Autodesk Inventor part; units mm, degrees
ref_plane "YZ Plane" through (0, 0, 0) normal (1, 0, 0) x (0, 1, 0)
ref_plane "XZ Plane" through (0, 0, 0) normal (0, 1, 0) x (-1, 0, 0)
ref_plane "XY Plane" through (0, 0, 0) normal (0, 0, 1) x (1, 0, 0)
sketch "Sketch1" plane through (0, 0, 0) normal (0, 1, 0) x (-1, 0, 0)
  line L0 (6, -3.4641) -> (0, -6.9282)
  line L1 (0, -6.9282) -> (-6, -3.4641)
  line L2 (-6, -3.4641) -> (-6, 3.4641)
  line L3 (-6, 3.4641) -> (0, 6.9282)
  line L4 (0, 6.9282) -> (6, 3.4641)
  line L5 (6, 3.4641) -> (6, -3.4641)
  circle A0 centre (0, 0) radius 2
  dimension "d0" = 6
  dimension "d1" = 4
extrude "Extrusion1" add sketch "Sketch1" along normal blind 6
sketch "Sketch2" plane through (0, 6, 0) normal (0, 1, 0) x (1, 0, 0)
  circle A0 centre (0, 0) radius 3
  circle A1 centre (0, 0) radius 5.5
  dimension "d4" = 6
  dimension "d5" = 11
extrude "Extrusion2" add sketch "Sketch2" along normal blind 12
sketch "Sketch3" plane through (0, 0, 0) normal (0, 0, 1) x (1, 0, 0)
  circle A0 centre (0, 15) radius 1.5
  line L0 (0, 0) -> (0, 6)
  line L1 (5.5, 18) -> (-5.5, 18)
  dimension "d16" = 3
  dimension "d44" = 0
  dimension "d45" = 3
extrude "Extrusion3" cut sketch "Sketch3" along normal mid plane 24
chamfer "Chamfer" distance 0.5 angle 45 4 edges at (2, 0, 0) (-3, 18, 0) (-1.5, 15.0054, -5.2915) (-1.5, 15.0054, 5.2915)
sketch "Sketch4" plane through (0, 0, 0) normal (1, 0, 0) x (0, 1, 0)
  line L0 (0, -3.4641) -> (0, -6.9282)
  line L1 (0, -6.9282) -> (0, -5.9282)
  line L2 (0, -6.9282) -> (1, -6.9282)
  line L3 (1, -6.9282) -> (0, -5.9282)
  line L4 (-6, 0) -> (36, 0)
  line L5 (0, -6.9282) -> (6, -6.9282)
  line L6 (6, -6.9282) -> (5, -6.9282)
  line L7 (6, -6.9282) -> (6, -5.9282)
  line L8 (6, -5.9282) -> (5, -6.9282)
  dimension "d31" = 1
  dimension "d32" = 1
  dimension "d36" = 1
  dimension "d37" = 1
revolve "Revolution" cut sketch "Sketch4" angle 360 about axis through (0, -10, 0) along (0, 1, 0)
thread "Thread1"
thread "Thread2"
thread "Thread3"
properties part number "6mmID_30mmL_hex_adapter"
Part model, mm, in its own coordinate system. A direction names the side the tool comes from. Coordinates: 2 decimals unless noted, no trailing zeros. Write each loop counter-clockwise with the first axis right and the second up, starting at its lowest first coordinate (ties: lowest second). Pieces come first, ordered by that corner, then holes.
Item 1: Mould opens along Z. For faces 3 (the face through (2.96, 2.96, -5.22)), 4 (the face through (1.61, 11.67, 2.53)), 5 (the face through (-4, 6, -4)), 6 (the face through (-1, 6, -2)) say: released by +Z, released by -Z, zero draft, split by the parting line, or undercut.
Item 2: Which spindle directions (+Z, -Z, +X, -X, +Y, -Y) get a long thin tool onto all of the face, cutting with end or side? Do faces 1 (the face through (1.43, 15.45, -3.78)), 2 (the face through (2.5, 11.9, -4.9)). Say none if no direction does.
Item 3: Slice it at C-C (x = -0.5). Count the separate pieces of the cut face and the enclosed holes in it, and give its area (3 significant figures).
Item 4: Pin check, flat tips, straight feed: pin 1 (3.5 mm diameter, centred on x = 0, z = 0, fed in from -Y); pin 2 (1.8 mm diameter, centred on x = 1, z = 1.5, fed in from +Y); pin 3 (1 mm diameter, centred on y = 7.5, z = -4, fed in from +X); pin 4 (5 mm diameter, centred on x = 2, y = 11.5, fed in from +Z). Stop position of each tip, or through.
Item 5: Slice it at B-B (y = 2.5). Write the cut outline in (x, z).
Item 6: Slice it at D-D (y = 11.5). Write the cut outline in (x, z), and give its area (3 significant figures).
Item 7: Slice it at A-A (z = 0). Write the cut outline in (x, y), and give its area (3 significant figures).
Item 8: Probe line 1 (Z direction, x = 0, y = 12); line 2 (Y direction, x = 0, z = 3.6); line 3 (Z direction, x = -1, y = 11). List the from-to ranges inside material, lowest first.
Results found:
1. face 3: released by -Z
1. face 4: undercut
1. face 5: zero draft
1. face 6: undercut
2. face 1: +Z, -Z
2. face 2: +Y
3. separate pieces: 4
3. enclosed holes: 0
3. area: 101 mm2
4. pin 1: passes through
4. pin 2: stops at y = 6
4. pin 3: stops at x = 4.24
4. pin 4: stops at z = 5.5
5. outline: (-6, -3.46) - (0, -6.93) - (6, -3.46) - (6, 3.46) - (0, 6.93) - (-6, 3.46) - close; hole circle Ø4 at (0, 0)
6. outline: circle Ø11 at (0, 0); hole circle Ø6 at (0, 0)
6. area: 66.8 mm2
7. outline: (-6, 0.07) - (-5.93, 0) - (-2.5, 0) - (-2, 0.5) - (-2, 6) - (-3, 6) - (-3, 17.5) - (-3.5, 18) - (-5.5, 18) - (-5.5, 6) - (-5.93, 6) - (-6, 5.93) - close; (2, 0.5) - (2.5, 0) - (5.93, 0) - (6, 0.07) - (6, 5.93) - (5.93, 6) - (5.5, 6) - (5.5, 18) - (3.5, 18) - (3, 17.5) - (3, 6) - (2, 6) - close
7. area: 107 mm2
8. line 1: z = -5.5 to -3, 3 to 5.5
8. line 2: y = 0 to 13.5, 16.5 to 18
8. line 3: z = -5.41 to -2.83, 2.83 to 5.41
